The model under review builds one solid part; all positions refer to its coordinate system, in mm. Face numbers are marked on the shaded views. A direction names the side the tool comes from. Round coordinates to 2 decimals unless told otherwise and drop trailing zeros. Loops run counter-clockwise (first coordinate to the right, second up) from the corner with the lowest first, then second, coordinate; pieces in that order, holes last. Notation, with made-up numbers: M -14,15.5 L 24,15.5 A22 cw 24,52.5 Z; hole C 48.5,43 d9. An arc over 180 degrees is marked long. Return JSON: item names as keys, results as strings. Group by question number.
Q1. Consider section A-A (z = 0). State the section outline as (x, y) points, and give its area (3 significant figures).
Q2. To check wall thickness, follow line 1 along X through (y, z) = (-2.25, 0); line 2 along X through (y, z) = (1, 0) (3 decimals); line 3 along X through (y, z) = (-4, -4). State the ranges of each line that lie inside material, in increasing order.
Q3. For the marked faces 1, 2 and 3, list the 3-axis set-ups (+Z, -Z, +X, -X, +Y, -Y) from which the entire face can be reached by the end or side of a thin tool; tool diameter is ignored.
Q4. Consider section C-C (y = 4.75). State the section outline as (x, z) points.
Q5. Clearance check with flat-ended pins moving along their axes: pin 1 Ø12 at (x, z) = (11.5, -20) entering from +Y; pin 2 Ø5 at (y, z) = (-1, 4.5) entering from -X; pin 3 Ø12 at (x, z) = (18.5, -4) entering from +Y. State where each tip first meets the part, or that it passes through.
Q6. Consider section B-B (y = -1). State the section outline as (x, z) points (3 decimals).
from build123d import *

# Parameters (mm, degrees)
CORTAR_EXTRUIR1_DEPTH = 45.022721406
CROQUIS4_R            = 2
CORTAR_EXTRUIR2_DEPTH = 45.022721406


with BuildPart() as part:
    # Croquis2 → Revolución1 (revolve)
    with BuildSketch(Plane(origin=(0, 0, 0), x_dir=(0, 0, -1), z_dir=(1, 0, 0))):
        Polygon((0, -8), (0, 8), (3, 8), (29, -8), align=None)
    revolve(axis=Axis((0, -8, 0), (0, 1, 0)))

    # Croquis3 → Cortar-Extruir1 (cut, through all)
    with BuildSketch(Plane(origin=(0, 8, 0), x_dir=(1, 0, 0), z_dir=(0, 1, 0))):
        with BuildLine():
            Line((0, 3), (0, 40.325375613))
            Line((0, 40.325375613), (-47.550667512, 40.325375613))
            Line((-47.550667512, 40.325375613), (-47.550667512, -39.963713052))
            Line((-47.550667512, -39.963713052), (0, -39.963713052))
            Line((0, -39.963713052), (0, -3))
            ThreePointArc((0, -3), (-3, 0), (0, 3))
        make_face()
    extrude(amount=-CORTAR_EXTRUIR1_DEPTH, mode=Mode.SUBTRACT)

    # Croquis4 → Cortar-Extruir2 (cut, through all)
    with BuildSketch(Plane(origin=(0, 8, 0), x_dir=(1, 0, 0), z_dir=(0, 1, 0))):
        with Locations(Location((0, 0, 0), (0, 0, 270))):
            Circle(CROQUIS4_R)
    extrude(amount=-CORTAR_EXTRUIR2_DEPTH, mode=Mode.SUBTRACT)


solid = part.part
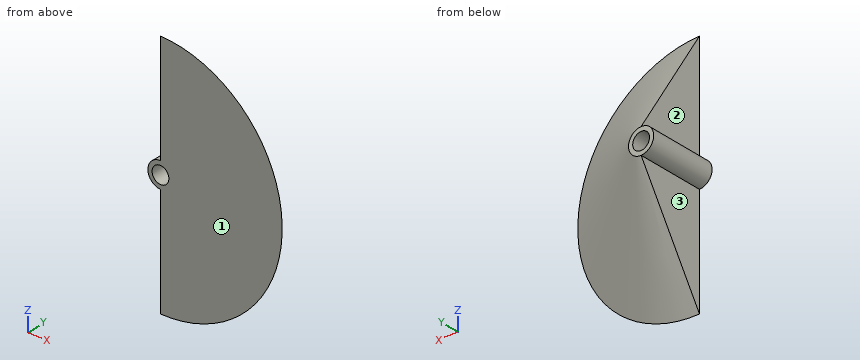
Values:
{
 "1": {"outline": "M -3,-8 L -2,-8 L -2,8 L -3,8 Z; M 2,-8 L 29,-8 L 3,8 L 2,8 Z", "area": "240 mm2"},
 "2": {"line 1": "x = -3 to -2, 2 to 19.66", "line 2": "x = -3 to -2, 2 to 14.375", "line 3": "x = 0 to 22.14"},
 "3": {"face 1": "+Z, -Z, +X, -X, -Y", "face 2": "+Z, -X, +Y, -Y", "face 3": "-Z, -X, +Y, -Y"},
 "4": {"outline": "M 0,-8.28 A8.28 ccw 0,8.28 L 0,3 A3 ccw 0,-3 Z; hole C 0,0 d4"},
 "5": {"pin 1": "stops at y = -0.66", "pin 2": "stops at x = -2.24", "pin 3": "stops at y = 1.89"},
 "6": {"outline": "M 0,-17.625 A17.625 ccw 0,17.625 L 0,3 A3 ccw 0,-3 Z; hole C 0,0 d4"}
}
